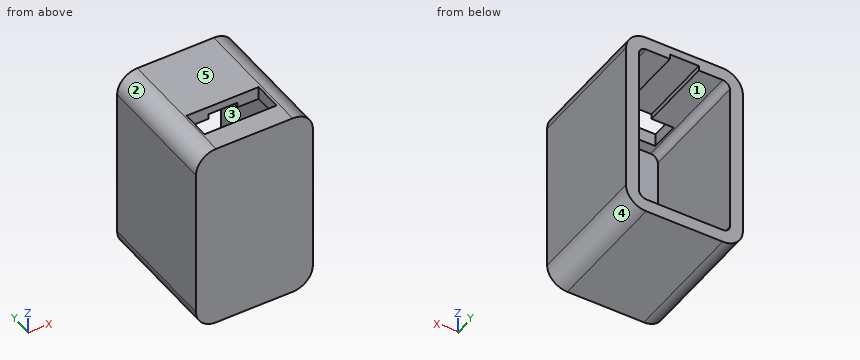
from build123d import *

# Parameters (mm, degrees)
BOSS_EXTRUDE1_DEPTH = 16
BOSS_EXTRUDE2_START = 1.5
BOSS_EXTRUDE2_DEPTH = 1.5
SKETCH3_W           = 10
SKETCH3_H           = 4
CUT_EXTRUDE1_DEPTH  = 2.5
SKETCH5_W           = 4
SKETCH5_H           = 1.4
CUT_EXTRUDE2_DEPTH  = 14


with BuildPart() as part:
    # Sketch1 → Boss-Extrude1 (new body)
    with BuildSketch(Plane(origin=(0, 0, 0), x_dir=(1, 0, 0), z_dir=(0, 1, 0))):
        with BuildLine():
            Line((-5.25, 13.3), (5.35, 13.3))
            ThreePointArc((5.35, 13.3), (7.329898987, 12.479898987), (8.15, 10.5))
            Line((8.15, 10.5), (8.15, -10.4))
            ThreePointArc((8.15, -10.4), (7.329898987, -12.379898987), (5.35, -13.2))
            Line((5.35, -13.2), (-5.25, -13.2))
            ThreePointArc((-5.25, -13.2), (-7.229898987, -12.379898987), (-8.05, -10.4))
            Line((-8.05, -10.4), (-8.05, 10.5))
            ThreePointArc((-8.05, 10.5), (-7.229898987, 12.479898987), (-5.25, 13.3))
        make_face()
        with BuildLine():
            Line((-5.25, 11.5), (5.35, 11.5))
            ThreePointArc((5.35, 11.5), (6.057106781, 11.207106781), (6.35, 10.5))
            Line((6.35, 10.5), (6.35, -10.4))
            ThreePointArc((6.35, -10.4), (6.057106781, -11.107106781), (5.35, -11.4))
            Line((5.35, -11.4), (-5.25, -11.4))
            ThreePointArc((-5.25, -11.4), (-5.957106781, -11.107106781), (-6.25, -10.4))
            Line((-6.25, -10.4), (-6.25, 10.5))
            ThreePointArc((-6.25, 10.5), (-5.957106781, 11.207106781), (-5.25, 11.5))
        make_face(mode=Mode.SUBTRACT)
    extrude(amount=BOSS_EXTRUDE1_DEPTH)

    # Sketch2 → Boss-Extrude2 (add)
    with BuildSketch(Plane.XZ.offset(BOSS_EXTRUDE2_START)):
        with BuildLine():
            Line((-5.25, 13.2), (5.35, 13.2))
            ThreePointArc((5.35, 13.2), (7.329898987, 12.379898987), (8.15, 10.4))
            Line((8.15, 10.4), (8.15, -10.5))
            ThreePointArc((8.15, -10.5), (7.329898987, -12.479898987), (5.35, -13.3))
            Line((5.35, -13.3), (-5.25, -13.3))
            ThreePointArc((-5.25, -13.3), (-7.229898987, -12.479898987), (-8.05, -10.5))
            Line((-8.05, -10.5), (-8.05, 10.4))
            ThreePointArc((-8.05, 10.4), (-7.229898987, 12.379898987), (-5.25, 13.2))
        make_face()
    extrude(amount=-BOSS_EXTRUDE2_DEPTH)

    # Sketch3 → Cut-Extrude1 (cut)
    with BuildSketch(Plane.XY.offset(13.2)):
        with Locations((0.0109375, 3.5)):
            Rectangle(SKETCH3_W, SKETCH3_H)
    extrude(amount=-CUT_EXTRUDE1_DEPTH, mode=Mode.SUBTRACT)

    # Sketch5 → Cut-Extrude2 (cut)
    with BuildSketch(Plane(origin=(0, 16, 0), x_dir=(1, 0, 0), z_dir=(0, 1, 0))):
        with Locations((0.05, -11.4)):
            Rectangle(SKETCH5_W, SKETCH5_H)
    extrude(amount=-CUT_EXTRUDE2_DEPTH, mode=Mode.SUBTRACT)


solid = part.part
Can you work these out from the model? Positions are in its coordinate system, mm. Face numbers are marked on the shaded views. A direction names the side the tool comes from. Give positions to 0.01 mm unless a question says otherwise; leave off trailing zeros. Write each loop counter-clockwise with the first axis right and the second up, starting at its lowest first coordinate (ties: lowest second). Pieces come first, ordered by that corner, then holes. Notation, with made-up numbers: (72.25, 12.25) -> (110.25, 12.25) arc R12 ccw to (110.25, 22.25) -> close; hole circle Ø8 at (33.25, 8.5). An arc over 180 degrees is marked (long way). Answer as a JSON object with one key per item and string values. Group by question number.
Item 1: Suppose I cut it at C-C (z = -5.75). Please give me the cut outline in (x, y), plus the area to 3 significant figures.
Item 2: Please list where these lines run through material, in increasing order: line 1 (Z direction, x = 4, y = 13.75); line 2 (Z direction, x = 1.75, y = 14.25); line 3 (X direction, y = 11.25, z = 1.75). Write a range as [from, to].
Item 3: For the marked faces 1 and 2, which set-ups out of +Z, -Z, +X, -X, +Y, -Y let a thin tool reach every point of the face, with its end or its side?
Item 4: I'm going to push flat-ended pins straight in: P1, Ø1.5, axis at x = 5, z = -5.5, coming from the +Y side; P2, Ø0.6, axis at y = 13, z = 11.5, coming from the -X side; P3, Ø2, axis at y = 4, z = 12.5, coming from the +X side. Where does each tip first touch, or does it pass through?
Item 5: We'd pull the mould along X, two halves only. Please class the marked faces 3, 4 and 5: +X half, -X half, draft (parallel to the pull), parting line (faces both ways), or undercut.
Item 6: Suppose I cut it at B-B (x = 4.5). Please give me the cut outline in (y, z).
Item 7: Suppose I cut it at A-A (y = 0.5). Please give me the cut outline in (x, z).
Item 8: Suppose I cut it at D-D (y = 3.5). Please give me the cut outline in (x, z).
Findings:
{
 "1": {"outline": "(-8.05, -1.5) -> (8.15, -1.5) -> (8.15, 16) -> (6.35, 16) -> (6.35, 0) -> (-6.25, 0) -> (-6.25, 16) -> (-8.05, 16) -> close", "area": "81.9 mm²"},
 "2": {"line 1": "z = [-13.3, -11.5], [11.4, 13.2]", "line 2": "z = [-13.3, -11.5], [12.1, 13.2]", "line 3": "x = [-8.05, -6.25], [6.35, 8.15]"},
 "3": {"face 1": "+Y", "face 2": "+Z, -X, +Y, -Y"},
 "4": {"P1": "stops at y = 0", "P2": "stops at x = -7.93", "P3": "stops at x = 7.92"},
 "5": {"face 3": "undercut", "face 4": "+X half", "face 5": "draft"},
 "6": {"outline": "(-1.5, -13.3) -> (16, -13.3) -> (16, -11.5) -> (0, -11.5) -> (0, 11.4) -> (1.5, 11.4) -> (1.5, 13.2) -> (-1.5, 13.2) -> close; (5.5, 11.4) -> (16, 11.4) -> (16, 13.2) -> (5.5, 13.2) -> close"},
 "7": {"outline": "(-8.05, -10.5) arc R2.8 ccw to (-5.25, -13.3) -> (5.35, -13.3) arc R2.8 ccw to (8.15, -10.5) -> (8.15, 10.4) arc R2.8 ccw to (5.35, 13.2) -> (-5.25, 13.2) arc R2.8 ccw to (-8.05, 10.4) -> close; hole (-6.25, -10.5) arc R1 ccw to (-5.25, -11.5) -> (5.35, -11.5) arc R1 ccw to (6.35, -10.5) -> (6.35, 10.4) arc R1 ccw to (5.35, 11.4) -> (-5.25, 11.4) arc R1 ccw to (-6.25, 10.4) -> close"},
 "8": {"outline": "(-8.05, -10.5) arc R2.8 ccw to (-5.25, -13.3) -> (5.35, -13.3) arc R2.8 ccw to (8.15, -10.5) -> (8.15, 10.4) arc R2.8 ccw to (5.35, 13.2) -> (5.01, 13.2) -> (5.01, 11.4) -> (5.35, 11.4) arc R1 cw to (6.35, 10.4) -> (6.35, -10.5) arc R1 cw to (5.35, -11.5) -> (-5.25, -11.5) arc R1 cw to (-6.25, -10.5) -> (-6.25, 10.4) arc R1 cw to (-5.25, 11.4) -> (-4.99, 11.4) -> (-4.99, 13.2) -> (-5.25, 13.2) arc R2.8 ccw to (-8.05, 10.4) -> close"}
}
